```python
from build123d import *

# Parameters (mm, degrees)
SKETCH1_W           = 8.9916
SKETCH1_H           = 1.905
BOSS_EXTRUDE1_DEPTH = 4.445
SKETCH1_4_W         = 3.3528
SKETCH1_4_H         = 1.524
BOSS_EXTRUDE2_DEPTH = 4.445
SKETCH1_6_W         = 3.3528
SKETCH1_6_H         = 1.524
BOSS_EXTRUDE3_DEPTH = 4.445
SKETCH1_8_W         = 3.3528
SKETCH1_8_H         = 1.524
BOSS_EXTRUDE4_DEPTH = 4.445
SKETCH1_10_W        = 6.7056
SKETCH1_10_H        = 3.2766
BOSS_EXTRUDE5_DEPTH = 3.3528
SKETCH2_W           = 5.969
SKETCH2_H           = 5.969
CUT_EXTRUDE1_DEPTH  = 11.0109
CUT_EXTRUDE2_REACH  = 35.62
SKETCH3_R           = 2.0574


with BuildPart() as part:
    # Sketch1 → Boss-Extrude1 (new, symmetric)
    with BuildSketch(Plane.XY):
        with Locations((0, 4.2291)):
            Rectangle(SKETCH1_W, SKETCH1_H)
    extrude(amount=BOSS_EXTRUDE1_DEPTH, both=True)

    # Sketch1_4 → Revolve1 (revolve)
    with BuildSketch(Plane.XY):
        with Locations((-1.6764, 5.9436)):
            Rectangle(SKETCH1_4_W, SKETCH1_4_H)
    revolve(axis=Axis((0, 6.7056, 0), (0, -1, 0)))

    # Sketch1_5 → Boss-Extrude2 (add, symmetric)
    with BuildSketch(Plane.XY):
        Polygon((0, 8.6106), (-3.3528, 8.6106), (-4.4958, 8.6106), (-4.4958, 6.7056), (-3.3528, 6.7056), (0, 6.7056), (3.3528, 6.7056), (4.4958, 6.7056), (4.4958, 8.6106), (3.3528, 8.6106), align=None)
    extrude(amount=BOSS_EXTRUDE2_DEPTH, both=True)

    # Sketch1_6 → Revolve2 (revolve)
    with BuildSketch(Plane.XY):
        with Locations((-1.6764, 9.3726)):
            Rectangle(SKETCH1_6_W, SKETCH1_6_H)
    revolve(axis=Axis((0, 10.1346, 0), (0, -1, 0)))

    # Sketch1_7 → Boss-Extrude3 (add, symmetric)
    with BuildSketch(Plane.XY):
        Polygon((-3.3528, 19.0246), (-4.4958, 19.0246), (-4.4958, 10.1346), (-3.3528, 10.1346), (0, 10.1346), (3.3528, 10.1346), (4.4958, 10.1346), (4.4958, 19.0246), (3.3528, 19.0246), (0, 19.0246), align=None)
    extrude(amount=BOSS_EXTRUDE3_DEPTH, both=True)

    # Sketch1_8 → Revolve3 (revolve)
    with BuildSketch(Plane.XY):
        with Locations((-1.6764, 19.7866)):
            Rectangle(SKETCH1_8_W, SKETCH1_8_H)
    revolve(axis=Axis((0, 20.5486, 0), (0, -1, 0)))

    # Sketch1_9 → Boss-Extrude4 (add, symmetric)
    with BuildSketch(Plane.XY):
        Polygon((-4.4958, 20.5486), (-3.3528, 20.5486), (0, 20.5486), (3.3528, 20.5486), (4.4958, 20.5486), (4.4958, 33.02), (-4.4958, 33.02), align=None)
    extrude(amount=BOSS_EXTRUDE4_DEPTH, both=True)

    # Sketch1_10 → Boss-Extrude5 (add, symmetric)
    with BuildSketch(Plane.XY):
        with Locations((0, 1.6383)):
            Rectangle(SKETCH1_10_W, SKETCH1_10_H)
    extrude(amount=BOSS_EXTRUDE5_DEPTH, both=True)

    # Sketch2 → Cut-Extrude1 (cut)
    with BuildSketch(Plane(origin=(0, 33.02, 0), x_dir=(1, 0, 0), z_dir=(0, 1, 0))):
        Rectangle(SKETCH2_W, SKETCH2_H)
    extrude(amount=-CUT_EXTRUDE1_DEPTH, mode=Mode.SUBTRACT)

    # Sketch3 → Cut-Extrude2 (cut, up to next)
    with BuildSketch(Plane(origin=(0, 0, 0), x_dir=(-1, 0, 0), z_dir=(0, -1, 0)), mode=Mode.PRIVATE) as cut_extrude2_sk1:
        with Locations(Location((0, 0, 0), (0, 0, 90))):
            Circle(SKETCH3_R)
    cut_extrude2_tool1 = extrude(cut_extrude2_sk1.sketch, amount=-CUT_EXTRUDE2_REACH, mode=Mode.PRIVATE) & part.part
    add(cut_extrude2_tool1.solids().sort_by_distance((0, 0, 0))[0], mode=Mode.SUBTRACT)


solid = part.part
```
Verification items for the finished model (mm, model axes). A direction names the side the tool comes from. Give positions to 0.01 mm unless a question says otherwise; leave off trailing zeros. Order: outer loops, then holes, each group sorted by start corner. A loop starts at its lowest first (then second) coordinate and runs counter-clockwise, first axis right, second up. Notation, with made-up numbers: M 69,62.25 L 120,62.25 A25 ccw 120,80.25 Z; hole C 60,57 d4. An arc over 180 degrees is marked long. Return JSON: item names as keys, results as strings. Group by question number.
1) Section check A-A on y = 26. Record the cut outline in (x, z) (1 decimal).
2) Go/stop test with flat-tipped pins: pin 1 Ø5 at (x, z) = (-1.5, 0.5) entering from +Y; pin 2 Ø4.5 at (x, z) = (0, 0) entering from +Y; pin 3 Ø2.5 at (y, z) = (1, -0.5) entering from +X; pin 4 Ø1 at (y, z) = (6, 3) entering from -X. Record where each tip stops, or that it passes through.
3) Mould release check, pull along Z, two halves, no side actions. Record for faces 1 (the face through (0, 2, -3.353)), 2 (the face through (0, 27, 4.445)), 3 (the face through (2.984, 28, 0)): pulls with the +Z half, pulls with the -Z half, needs draft (parallel to the pull), parting line crosses it, or undercut.
4) Scan lines: line 1 (Y direction, x = -4, z = 2.5); line 2 (X direction, y = 4.75, z = 0); line 3 (Z direction, x = -1.5, y = 31) (1 decimal). Record each from-to range of solid material in increasing order.
5) Access from +Z, -Z, +X, -X, +Y, -Y to the whole of each face (thin tool, end or side, straight path). Record for faces 4 (the face through (0, 27, -4.445)), 5 (the face through (0, 28, -2.984)), 6 (the face through (-3.353, 2, 0)), 7 (the face through (-4.496, 4, 0)), 8 (the face through (0.727, 19.797, 3.273)).
Answer block:
{
 "1": {"outline": "M -4.5,-4.4 L 4.5,-4.4 L 4.5,4.4 L -4.5,4.4 Z; hole M -3,-3 L 3,-3 L 3,3 L -3,3 Z"},
 "2": {"pin 1": "stops at y = 33.02", "pin 2": "stops at y = 22.01", "pin 3": "stops at x = 3.35", "pin 4": "stops at x = -2.23"},
 "3": {"face 1": "pulls with the -Z half", "face 2": "pulls with the +Z half", "face 3": "undercut"},
 "4": {"line 1": "y = 3.28 to 5.18, 6.71 to 8.61, 10.13 to 19.02, 20.55 to 33.02", "line 2": "x = -4.5 to -2.06, 2.06 to 4.5", "line 3": "z = -4.4 to -3, 3 to 4.4"},
 "5": {"face 4": "-Z, +X, -X, +Y, -Y", "face 5": "+Y", "face 6": "+Z, -Z, -X, -Y", "face 7": "+Z, -Z, -X, +Y, -Y", "face 8": "none"}
}
